from build123d import *

# Parameters (mm, degrees)
F0_R     = 4.2
F1_DEPTH = 9.6
F2_R     = 1.5
F3_DEPTH = 19.051
F4_W     = 9.64414
F4_H     = 2
F5_DEPTH = 11.901


with BuildPart() as f1:
    # F0 (on Right) → F1 (new body)
    with BuildSketch(Plane.YZ):
        with BuildLine():
            Line((-9.525, 7.133328), (-9.525, -7.133328))
            ThreePointArc((-9.525, -7.133328), (-8.813863, -7.995362), (-8.025, -8.786887))
            ThreePointArc((-8.025, -8.786887), (0, -11.9), (8.025, -8.786887))
            ThreePointArc((8.025, -8.786887), (8.813863, -7.995362), (9.525, -7.133328))
            Line((9.525, -7.133328), (9.525, 7.133328))
            ThreePointArc((9.525, 7.133328), (0, 11.9), (-9.525, 7.133328))
        make_face()
        Circle(F0_R, mode=Mode.SUBTRACT)
        with BuildLine():
            ThreePointArc((8.025, -8.786887), (0, -11.9), (-8.025, -8.786887))
            Line((-8.025, -8.786887), (-8.025, -16.4))
            Line((-8.025, -16.4), (8.025, -16.4))
            Line((8.025, -16.4), (8.025, -8.786887))
        make_face()
    extrude(amount=F1_DEPTH)

    # F2 (on face) → F3 (cut, through all)
    with BuildSketch(Plane.XZ.offset(9.525)):
        with Locations((4.642159, 7.4)):
            Circle(F2_R)
    extrude(amount=-F3_DEPTH, mode=Mode.SUBTRACT)

    # F4 (on Top) → F5 (cut, through all)
    with BuildSketch(Plane.XY):
        with Locations((4.82207, 0)):
            Rectangle(F4_W, F4_H)
    extrude(amount=F5_DEPTH, mode=Mode.SUBTRACT)


solid = f1.part
Source: CAD feature listing. Evaluate the final solid. Frame: model axes, mm. A direction names the side the tool comes from. Give positions to 0.01 mm unless a question says otherwise; leave off trailing zeros. Write each loop counter-clockwise with the first axis right and the second up, starting at its lowest first coordinate (ties: lowest second). Pieces come first, ordered by that corner, then holes. Notation, with made-up numbers: M -16.75,61 L 34.25,61 A21 cw 34.25,80 Z; hole C 22,27.25 d11. An arc over 180 degrees is marked long. Return JSON: item names as keys, results as strings. Group by question number.
1) Pull-direction query (Y, two-part tool) for faces 4 (the face through (5, -8.025, -13)), 5 (the face through (4, 1, 9)), 6 (the face through (4.317, -5.322, 5.936)); classes: pulls with the +Y half, pulls with the -Y half, needs draft (parallel to the pull), parting line crosses it, or undercut.
2) Cut plane A-A, the plane y = -3.5. Output: boundary loops of the cut face in (x, z), plus the area to 3 significant figures.
3) Cut plane C-C, the plane x = 1.25. Output: boundary loops of the cut face in (y, z) (3 decimals), plus the area to 3 significant figures.
4) Cut plane D-D, the plane y = -7. Output: boundary loops of the cut face in (x, z), plus the area to 3 significant figures.
5) Material intervals for line 1 along X through (y, z) = (-6.25, 7.4); line 2 along Z through (x, y) = (4.5, -3); line 3 along Y through (x, z) = (4, 0) (3 decimals), sorted ascending. Write a range as [from, to].
6) Pin query (flat end, axial travel): P1, Ø1, axis at x = 5, y = -2, coming from the +Z side; P2, Ø3, axis at x = 5, y = 7.5, coming from the +Z side; P3, Ø1.5, axis at x = 8.5, z = -11, coming from the -Y side (3 decimals). Return the tip coordinate at first contact, or that it passes through.
7) Cut plane B-B, the plane z = 5.25. Output: boundary loops of the cut face in (x, y) (3 decimals).
8) Set-up query: faces 1 (the face through (5, 8.025, -13)), 2 (the face through (4, -1, 9)), 3 (the face through (9.6, 0, -5)). Return all of +Z, -Z, +X, -X, +Y, -Y with unobstructed straight access to the full face (end or side cutting, diameter ignored); none if empty.
Recorded:
{
 "1": {"face 4": "pulls with the -Y half", "face 5": "undercut", "face 6": "needs draft"},
 "2": {"outline": "M 0,-16.4 L 9.6,-16.4 L 9.6,-2.32 L 0,-2.32 Z; M 0,2.32 L 9.6,2.32 L 9.6,11.37 L 0,11.37 Z; hole C 4.64,7.4 d3", "area": "215 mm²"},
 "3": {"outline": "M -9.525,-7.133 A11.9 ccw -8.025,-8.787 L -8.025,-16.4 L 8.025,-16.4 L 8.025,-8.787 A11.9 ccw 9.525,-7.133 L 9.525,7.133 A11.9 ccw 1,11.858 L 1,4.079 A4.2 cw long -1,4.079 L -1,11.858 A11.9 ccw -9.525,7.133 Z", "area": "416 mm²"},
 "4": {"outline": "M 0,-16.4 L 9.6,-16.4 L 9.6,9.62 L 0,9.62 Z; hole C 4.64,7.4 d3", "area": "243 mm²"},
 "5": {"line 1": "x = [0, 3.14], [6.14, 9.6]", "line 2": "z = [-16.4, -2.94], [2.94, 5.91], [8.89, 11.52]", "line 3": "y = [-9.525, -4.2], [4.2, 9.525]"},
 "6": {"P1": "stops at z = 11.81", "P2": "stops at z = 10.28", "P3": "stops at y = -8.025"},
 "7": {"outline": "M 0,-9.525 L 9.6,-9.525 L 9.6,-1 L 0,-1 Z; M 0,1 L 9.6,1 L 9.6,9.525 L 0,9.525 Z"},
 "8": {"face 1": "-Z, +X, -X, +Y", "face 2": "+Z, +X, -X", "face 3": "+Z, -Z, +X, +Y, -Y"}
}
